Autodesk Inventor part; units mm, degrees
ref_plane "YZ Plane" through (0, 0, 0) normal (1, 0, 0) x (0, 1, 0)
ref_plane "XZ Plane" through (0, 0, 0) normal (0, 1, 0) x (-1, 0, 0)
ref_plane "XY Plane" through (0, 0, 0) normal (0, 0, 1) x (1, 0, 0)
sketch "スケッチ1" plane through (0, 0, 0) normal (0, 0, 1) x (1, 0, 0)
  circle A0 centre (0, 0) radius 5
  circle A1 centre (-20, 0) radius 1.6
  circle A2 centre (20, 0) radius 1.6
  circle A3 centre (-9.525, 0) radius 1.25
  circle A4 centre (9.525, 0) radius 1.25
  line L0 (-20, 0) -> (20, 0) construction
  arc A5 (-21, 3.873) -> (-21, -3.873) centre (-20, 0) ccw
  arc A6 (21, -3.873) -> (21, 3.873) centre (20, 0) ccw
  arc A7 (2.25, 8.7142) -> (-2.25, 8.7142) centre (0, 0) ccw
  arc A8 (-2.25, -8.7142) -> (2.25, -8.7142) centre (0, 0) ccw
  line L1 (-21, 3.873) -> (-2.25, 8.7142)
  line L2 (2.25, 8.7142) -> (21, 3.873)
  line L3 (21, -3.873) -> (2.25, -8.7142)
  line L4 (-2.25, -8.7142) -> (-21, -3.873)
  dimension "d0" = 10
  dimension "d1" = 3.2
  dimension "d2" = 3.2
  dimension "d3" = 40
  dimension "d4" = 20
  dimension "d5" = 2.5
  dimension "d6" = 2.5
  dimension "d7" = 19.05
  dimension "d8" = 9.525
  dimension "d9" = 4
  dimension "d10" = 4
  dimension "d11" = 9
  dimension "d12" = 9
extrude "押し出し1" add sketch "スケッチ1" along normal blind 3
properties part number "エンコーダマウント" material "ポリカーボネート、スモーク"
Geometry: final body of the model. Coordinates: model frame, mm. Coordinates: 2 decimals unless noted, no trailing zeros. Order: outer loops, then holes, each group sorted by start corner. A loop starts at its lowest first (then second) coordinate and runs counter-clockwise, first axis right, second up.
(1) Material intervals for probe 1 along Y at (x, z) = (0, 1.5); probe 2 along X at (y, z) = (-1.75, 2.2); probe 3 along Y at (x, z) = (10, 2.35), sorted ascending.
(2) Draft query along Y for faces 1 (the face through (-21.18, -1.08, 1.48)), 2 (the face through (0, 9, 1)), 3 (the face through (-24, 0, 1)). Return one class per face: pulls with the +Y half, pulls with the -Y half, needs draft (parallel to the pull), parting line crosses it, or undercut.
(3) Section query C-C (z = 0.9). Return the cut outline in (x, y) (3 decimals).
(4) Section query B-B (x = 0). Return the cut outline in (y, z), plus the area to 3 significant figures.
(5) Section query A-A (y = 0). Return the cut outline in (x, z) (3 decimals).
(6) Section query D-D (x = 20). Return the cut outline in (y, z).
(7) First-contact query: pin 1 (1.5 mm diameter, centred on y = -1, z = 1.5, fed in from +X); pin 2 (3.5 mm diameter, centred on x = -20, y = 0, fed in from +Z); pin 3 (2 mm diameter, centred on x = 9.525, y = 0, fed in from -Z). Flat tips, straight axial feed; report the tip coordinate or a pass-through.
Solution:
1. probe 1: y = -9 to -5, 5 to 9
1. probe 2: x = -23.6 to -4.68, 4.68 to 23.6
1. probe 3: y = -6.71 to -1.16, 1.16 to 6.71
2. face 1: undercut
2. face 2: pulls with the +Y half
2. face 3: parting line crosses it
3. outline: (-21, -3.873) - (-2.25, -8.714) arc R9 ccw to (2.25, -8.714) - (21, -3.873) arc R4 ccw to (21, 3.873) - (2.25, 8.714) arc R9 ccw to (-2.25, 8.714) - (-21, 3.873) arc R4 ccw to start; hole circle Ø3.2 at (-20, 0); hole circle Ø2.5 at (-9.525, 0); hole circle Ø10 at (0, 0); hole circle Ø2.5 at (9.525, 0); hole circle Ø3.2 at (20, 0)
4. outline: (-9, 0) - (-5, 0) - (-5, 3) - (-9, 3) - close; (5, 0) - (9, 0) - (9, 3) - (5, 3) - close
4. area: 24.0 mm2
5. outline: (-24, 0) - (-21.6, 0) - (-21.6, 3) - (-24, 3) - close; (-18.4, 0) - (-10.775, 0) - (-10.775, 3) - (-18.4, 3) - close; (-8.275, 0) - (-5, 0) - (-5, 3) - (-8.275, 3) - close; (5, 0) - (8.275, 0) - (8.275, 3) - (5, 3) - close; (10.775, 0) - (18.4, 0) - (18.4, 3) - (10.775, 3) - close; (21.6, 0) - (24, 0) - (24, 3) - (21.6, 3) - close
6. outline: (-4.13, 0) - (-1.6, 0) - (-1.6, 3) - (-4.13, 3) - close; (1.6, 0) - (4.13, 0) - (4.13, 3) - (1.6, 3) - close
7. pin 1: stops at x = 23.99
7. pin 2: stops at z = 3
7. pin 3: passes through
